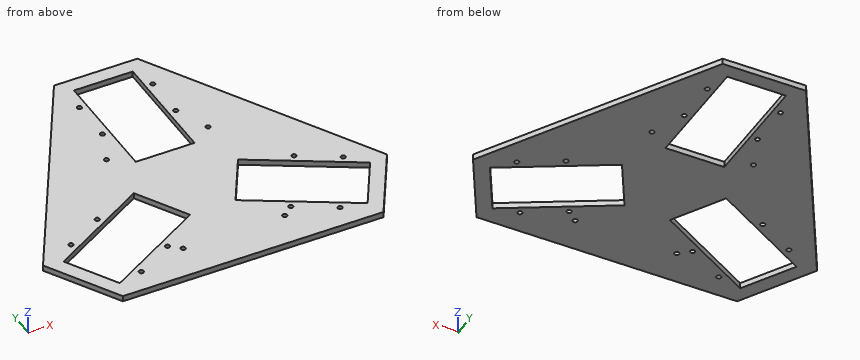
```python
from build123d import *

# Parameters (mm, degrees)
SKETCH_1_R      = 1.6
SKETCH_1_W      = 40.5
SKETCH_1_H      = 80.5
EXTRUDE_1_DEPTH = 4


with BuildPart() as part:
    # ｽｹｯﾁ1 → ﾎﾞｽ - 押し出し1 (new body)
    with BuildSketch(Plane.XY):
        Polygon((-28.723175892, 120.25), (28.723175892, 120.25), (118.501142751, -35.25), (89.777966859, -85), (-89.777966859, -85), (-118.501142751, -35.25), align=None)
        with Locations((25.25, 93.660254038)):
            Circle(SKETCH_1_R, mode=Mode.SUBTRACT)
        with Locations((25.25, 63.660254038)):
            Circle(SKETCH_1_R, mode=Mode.SUBTRACT)
        with Locations((-25.25, 63.660254038)):
            Circle(SKETCH_1_R, mode=Mode.SUBTRACT)
        with Locations((-25.25, 93.660254038)):
            Circle(SKETCH_1_R, mode=Mode.SUBTRACT)
        with Locations((68.487159322, -68.697268464)):
            Circle(SKETCH_1_R, mode=Mode.SUBTRACT)
        with Locations((93.737159322, -24.962985573)):
            Circle(SKETCH_1_R, mode=Mode.SUBTRACT)
        with Locations((67.756397208, -9.962985573)):
            Circle(SKETCH_1_R, mode=Mode.SUBTRACT)
        with Locations((42.506397208, -53.697268464)):
            Circle(SKETCH_1_R, mode=Mode.SUBTRACT)
        with Locations((-93.737159322, -24.962985573)):
            Circle(SKETCH_1_R, mode=Mode.SUBTRACT)
        with Locations((-68.487159322, -68.697268464)):
            Circle(SKETCH_1_R, mode=Mode.SUBTRACT)
        with Locations((-42.506397208, -53.697268464)):
            Circle(SKETCH_1_R, mode=Mode.SUBTRACT)
        with Locations((-67.756397208, -9.962985573)):
            Circle(SKETCH_1_R, mode=Mode.SUBTRACT)
        with Locations((-35, 40)):
            Circle(SKETCH_1_R, mode=Mode.SUBTRACT)
        with Locations((35, 40)):
            Circle(SKETCH_1_R, mode=Mode.SUBTRACT)
        with Locations((35, -60)):
            Circle(SKETCH_1_R, mode=Mode.SUBTRACT)
        with Locations((-35, -60)):
            Circle(SKETCH_1_R, mode=Mode.SUBTRACT)
        with Locations((0, 70)):
            Rectangle(SKETCH_1_W, SKETCH_1_H, mode=Mode.SUBTRACT)
        Polygon((105.604300767, -37.587985573), (85.354300767, -72.662014427), (15.639255763, -32.412014427), (35.889255763, 2.662014427), align=None, mode=Mode.SUBTRACT)
        Polygon((-85.354300767, -72.662014427), (-105.604300767, -37.587985573), (-35.889255763, 2.662014427), (-15.639255763, -32.412014427), align=None, mode=Mode.SUBTRACT)
    extrude(amount=EXTRUDE_1_DEPTH)


solid = part.part
```
For this review, take the finished solid that the model builds, in its own axes (mm). Round coordinates to 2 decimals unless told otherwise and drop trailing zeros. Write each loop counter-clockwise with the first axis right and the second up, starting at its lowest first coordinate (ties: lowest second). Pieces come first, ordered by that corner, then holes. Notation, with made-up numbers: M -23,55 L -8,55 A13 ccw -8,75 Z; hole C 10.25,-3 d6. An arc over 180 degrees is marked long. One line per item, written item: value. Start each with the question number.
(1) We need section B-B (x = 55). Give the boundary of the cut face in (y, z).
(2) Insertion check: pin 1 (2 mm diameter, centred on y = 70.5, z = 0.5, fed in from +X); pin 2 (2 mm diameter, centred on y = 82, z = 3, fed in from +X); pin 3 (1.5 mm diameter, centred on y = -21, z = 2, fed in from +X). Each pin has a flat end and moves straight along its axis. Give the tip position at first contact, or say it passes through.
(3) We need section C-C (z = 1.3). Count the separate pieces of the cut face and the enclosed holes in it, and give its area (3 significant figures).
(4) Wall thickness on line 1 (X direction, y = 41, z = 1.3); line 2 (X direction, y = -59.5, z = 0.4); line 3 (X direction, y = 40.5, z = 0.4): over which ranges is each line inside the solid? List them lowest first.
(5) We need section A-A (y = 33). Give the boundary of the cut face in (x, z).
Result:
1. outline: M -85,0 L -55.14,0 L -55.14,4 L -85,4 Z; M -8.37,0 L 74.74,0 L 74.74,4 L -8.37,4 Z
2. pin 1: x = 58.02
2. pin 2: x = 51.38
2. pin 3: x = 110.71
3. separate pieces: 1
3. enclosed holes: 19
3. area: 23,300 mm²
4. line 1: -74.48 to -36.25, -33.75 to -20.25, 20.25 to 33.75, 36.25 to 74.48
4. line 2: -104.5 to -92.95, -62.56 to -36.52, -33.48 to 33.48, 36.52 to 62.56, 92.95 to 104.5
4. line 3: -74.77 to -36.52, -33.48 to -20.25, 20.25 to 33.48, 36.52 to 74.77
5. outline: M -79.1,0 L -20.25,0 L -20.25,4 L -79.1,4 Z; M 20.25,0 L 79.1,0 L 79.1,4 L 20.25,4 Z
